from build123d import *

# Parameters (mm, degrees)
F1_DEPTH = 30
F2_R     = 10.5
F3_DEPTH = 25
F2_R_2   = 15
F4_DEPTH = 25


with BuildPart() as f1:
    # F0 (on Top) → F1 (new body)
    with BuildSketch(Plane.XY):
        with BuildLine():
            ThreePointArc((8.8575914058, 27), (4.5402897901, 25.5062154657), (0, 25))
            ThreePointArc((0, 25), (-4.5402897901, 25.5062154657), (-8.8575914058, 27))
            Line((-8.8575914058, 27), (-87.5, 27))
            ThreePointArc((-87.5, 27), (-87.5403243724, 25.9967636098), (-87.6610373207, 25))
            Line((-87.6610373207, 25), (-10.1980390272, 25))
            ThreePointArc((-10.1980390272, 25), (0, -27), (10.1980390272, 25))
            Line((10.1980390272, 25), (87.6610373207, 25))
            ThreePointArc((87.6610373207, 25), (87.5403243724, 25.9967636098), (87.5, 27))
            Line((87.5, 27), (8.8575914058, 27))
        make_face()
        with BuildLine():
            ThreePointArc((0, 25), (17.6776695297, 17.6776695297), (25, 0))
            ThreePointArc((25, 0), (-17.6776695297, -17.6776695297), (0, 25))
        make_face(mode=Mode.SUBTRACT)
        with BuildLine():
            ThreePointArc((112.5, 27), (100, 39.5), (87.5, 27))
            Line((87.5, 27), (100, 27))
            Line((100, 27), (100, 25))
            Line((100, 25), (87.6610373207, 25))
            ThreePointArc((87.6610373207, 25), (101.0032363902, 14.5403243724), (112.5, 27))
        make_face()
        with BuildLine():
            Line((100, 27), (87.5, 27))
            ThreePointArc((87.5, 27), (87.5403243724, 25.9967636098), (87.6610373207, 25))
            Line((87.6610373207, 25), (100, 25))
            Line((100, 25), (100, 27))
        make_face()
        with BuildLine():
            Line((-100, 27), (-87.5, 27))
            ThreePointArc((-87.5, 27), (-112.4596756276, 28.0032363902), (-87.6610373207, 25))
            Line((-87.6610373207, 25), (-100, 25))
            Line((-100, 25), (-100, 27))
        make_face()
        with BuildLine():
            ThreePointArc((-8.8575914058, 27), (-4.5402897901, 25.5062154657), (0, 25))
            ThreePointArc((0, 25), (4.5402897901, 25.5062154657), (8.8575914058, 27))
            Line((8.8575914058, 27), (0, 27))
            Line((0, 27), (-8.8575914058, 27))
        make_face()
        with BuildLine():
            ThreePointArc((20.6142313778, 45.6142313778), (-11.0080447085, 63.0432154846), (-8.8575914058, 27))
            Line((-8.8575914058, 27), (0, 27))
            Line((0, 27), (8.8575914058, 27))
            ThreePointArc((8.8575914058, 27), (17.4289841068, 34.6061866693), (20.6142313778, 45.6142313778))
        make_face()
        with BuildLine():
            ThreePointArc((-87.6610373207, 25), (-87.5403243724, 25.9967636098), (-87.5, 27))
            Line((-87.5, 27), (-100, 27))
            Line((-100, 27), (-100, 25))
            Line((-100, 25), (-87.6610373207, 25))
        make_face()
    extrude(amount=F1_DEPTH)

    # F2 (on face) → F3 (cut)
    with BuildSketch(Plane.XY.offset(30)):
        with Locations((100, 27)):
            Circle(F2_R)
        with Locations((-100, 27)):
            Circle(F2_R)
    extrude(amount=-F3_DEPTH, mode=Mode.SUBTRACT)

    # F2 (on face) → F4 (cut)
    with BuildSketch(Plane.XY.offset(30)):
        with Locations((0, 45.6142313778)):
            Circle(F2_R_2)
    extrude(amount=-F4_DEPTH, mode=Mode.SUBTRACT)


solid = f1.part
CAD build for the part. Positions are in the model's coordinates, mm. A direction names the side the tool comes from. Coordinates: 2 decimals unless noted, no trailing zeros. Order: outer loops, then holes, each group sorted by start corner. A loop starts at its lowest first (then second) coordinate and runs counter-clockwise, first axis right, second up. Notation, with made-up numbers: (-31.5, -28) -> (-21.5, -28) arc R17 cw to (-21.5, -7) -> close; hole circle Ø9 at (85.5, 43). An arc over 180 degrees is marked (long way). Answer in a Markdown table with one row per item.
1) Band-saw the part on D-D (y = 22). List the corners of the cut face in (x, z), and give its area (3 significant figures).
Check values:
| item | result |
|---|---|
| outline | (-111.46, 0) -> (-88.54, 0) -> (-88.54, 30) -> (-90.77, 30) -> (-90.77, 5) -> (-109.23, 5) -> (-109.23, 30) -> (-111.46, 30) -> close; (-15.65, 0) -> (-11.87, 0) -> (-11.87, 30) -> (-15.65, 30) -> close; (11.87, 0) -> (15.65, 0) -> (15.65, 30) -> (11.87, 30) -> close; (88.54, 0) -> (111.46, 0) -> (111.46, 30) -> (109.23, 30) -> (109.23, 5) -> (90.77, 5) -> (90.77, 30) -> (88.54, 30) -> close |
| area | 678 mm2 |
2) Band-saw the part on B-B (x = -100). List the corners of the cut face in (y, z), and give its area (3 significant figures).
Check values:
| item | result |
|---|---|
| outline | (14.5, 0) -> (39.5, 0) -> (39.5, 30) -> (37.5, 30) -> (37.5, 5) -> (16.5, 5) -> (16.5, 30) -> (14.5, 30) -> close |
| area | 225 mm2 |
3) Mould opens along Y. For faces 4 (the face through (0, 46, 5)), 5 (the face through (-1.953, 60.487, 17.675)), 6 (the face through (-1, 30, 0)), 7 (the face through (-112.405, 28.536, 14.79)) say: pulls with the +Y half, pulls with the -Y half, needs draft (parallel to the pull), parting line crosses it, or undercut.
Check values:
| item | result |
|---|---|
| face 4 | undercut |
| face 5 | undercut |
| face 6 | needs draft |
| face 7 | parting line crosses it |
4) Band-saw the part on A-A (z = 19). List the corners of the cut face in (x, y), and give its area (3 significant figures).
Check values:
| item | result |
|---|---|
| outline | (-87.66, 25) -> (-10.2, 25) arc R27 ccw (long way) to (10.2, 25) -> (87.66, 25) arc R12.5 ccw (long way) to (87.5, 27) -> (8.86, 27) arc R20.61 ccw (long way) to (-8.86, 27) -> (-87.5, 27) arc R12.5 ccw (long way) to start; hole circle Ø21 at (-100, 27); hole circle Ø50 at (0, 0); hole circle Ø30 at (0, 45.61); hole circle Ø21 at (100, 27) |
| area | 1,540 mm2 |
5) Band-saw the part on C-C (y = -10.5). List the corners of the cut face in (x, z).
Check values:
| item | result |
|---|---|
| outline | (-24.87, 0) -> (-22.69, 0) -> (-22.69, 30) -> (-24.87, 30) -> close; (22.69, 0) -> (24.87, 0) -> (24.87, 30) -> (22.69, 30) -> close |
6) Flat gauge pins, fed straight in: P1, Ø19, axis at x = 100, y = 27, coming from the +Z side; P2, Ø15, axis at x = 32.5, z = 15.5, coming from the -Y side; P3, Ø24, axis at x = 0, y = 45.61, coming from the -Z side; P4, Ø2, axis at x = 63.5, z = 13, coming from the -Y side. Where does each tip first touch, or does it go through?
Check values:
| item | result |
|---|---|
| P1 | z = 5 |
| P2 | y = -10.2 |
| P3 | z = 0 |
| P4 | y = 25 |
7) Which spindle directions (+Z, -Z, +X, -X, +Y, -Y) get a long thin tool onto all of the face, cutting with end or side? Do faces 1 (the face through (-1, 27, 30)), 2 (the face through (-49, 25, 15)), 3 (the face through (100, 27, 5)). Say none if no direction does.
Check values:
| item | result |
|---|---|
| face 1 | +Z, +X, -X, +Y, -Y |
| face 2 | +Z, -Z |
| face 3 | +Z |
8) Drill centre lines: line 1 (X direction, y = 1, z = 9); line 2 (X direction, y = 35, z = 17.5); line 3 (Y direction, x = 67.5, z = 13). Where is each one in solid material? Low to high.
Check values:
| item | result |
|---|---|
| line 1 | -26.98 to -24.98, 24.98 to 26.98 |
| line 2 | -109.6 to -106.8, -93.2 to -90.4, -17.67 to -10.6, 10.6 to 17.67, 90.4 to 93.2, 106.8 to 109.6 |
| line 3 | 25 to 27 |
